from build123d import *

# Parameters (mm, degrees)
SKETCH_1_W           = 25.4
SKETCH_1_H           = 25.4
EXTRUDE_1_DEPTH      = 400.8
SKETCH_1_3_W         = 21.4
SKETCH_1_3_H         = 21.4
CUT_EXTRUDE_1_DEPTH  = 402.202218339
SKETCH_2_R           = 2.15
CUT_EXTRUDE_2_DEPTH  = 3
SKETCH_3_R           = 2.15
CUT_EXTRUDE_3_DEPTH  = 3
SKETCH_4_R           = 2.15
CUT_EXTRUDE_4_DEPTH  = 3
SKETCH_5_R           = 2.149999993
CUT_EXTRUDE_5_DEPTH  = 5
SKETCH_6_R           = 2.15
CUT_EXTRUDE_6_DEPTH  = 5
SKETCH_7_R           = 2.15
CUT_EXTRUDE_7_DEPTH  = 5
SKETCH_8_R           = 2.15
CUT_EXTRUDE_8_DEPTH  = 5
SKETCH_9_R           = 2.15
CUT_EXTRUDE_9_DEPTH  = 5
SKETCH_10_R          = 2.15
CUT_EXTRUDE_10_DEPTH = 5
SKETCH_12_R          = 2.15
CUT_EXTRUDE_11_DEPTH = 5
SKETCH_13_R          = 2.15
CUT_EXTRUDE_12_DEPTH = 5
SKETCH_14_R          = 2.15
CUT_EXTRUDE_13_DEPTH = 5
SKETCH_15_R          = 2.15
CUT_EXTRUDE_14_DEPTH = 5
SKETCH_16_R          = 2.5
CUT_EXTRUDE_15_DEPTH = 10
SKETCH_17_R          = 2.5
CUT_EXTRUDE_16_DEPTH = 10


with BuildPart() as part:
    # Sketch 1 → Extrude 1 (new body)
    with BuildSketch(Plane.XY):
        Rectangle(SKETCH_1_W, SKETCH_1_H)
    extrude(amount=EXTRUDE_1_DEPTH)

    # Sketch 1_3 → Cut-Extrude 1 (cut, through all)
    with BuildSketch(Plane.XY):
        Rectangle(SKETCH_1_3_W, SKETCH_1_3_H)
    extrude(amount=CUT_EXTRUDE_1_DEPTH, mode=Mode.SUBTRACT)

    # Sketch 2 → Cut-Extrude 2 (cut)
    with BuildSketch(Plane(origin=(12.7, 0, 0), x_dir=(0, 0, -1), z_dir=(1, 0, 0))):
        with Locations(Location((-43.1, 0, 0), (0, 0, 90))):
            Circle(SKETCH_2_R)
        with Locations(Location((-67.6, 0, 0), (0, 0, 90))):
            Circle(SKETCH_2_R)
    extrude(amount=-CUT_EXTRUDE_2_DEPTH, mode=Mode.SUBTRACT)

    # Sketch 3 → Cut-Extrude 3 (cut)
    with BuildSketch(Plane.XZ.offset(12.7)):
        with Locations(Location((0, 43.1, 0), (0, 0, 270))):
            Circle(SKETCH_3_R)
        with Locations(Location((0, 67.6, 0), (0, 0, 270))):
            Circle(SKETCH_3_R)
    extrude(amount=-CUT_EXTRUDE_3_DEPTH, mode=Mode.SUBTRACT)

    # Sketch 4 → Cut-Extrude 4 (cut)
    with BuildSketch(Plane(origin=(12.7, 0, 0), x_dir=(0, 0, -1), z_dir=(1, 0, 0))):
        with Locations(Location((-104.95, 0, 0), (0, 0, 90))):
            Circle(SKETCH_4_R)
    extrude(amount=-CUT_EXTRUDE_4_DEPTH, mode=Mode.SUBTRACT)

    # Sketch 5 → Cut-Extrude 5 (cut)
    with BuildSketch(Plane.XZ.offset(12.7)):
        with Locations(Location((0, 104.95, 0), (0, 0, 270))):
            Circle(SKETCH_5_R)
    extrude(amount=-CUT_EXTRUDE_5_DEPTH, mode=Mode.SUBTRACT)

    # Sketch 6 → Cut-Extrude 6 (cut)
    with BuildSketch(Plane(origin=(12.7, 0, 0), x_dir=(0, 0, -1), z_dir=(1, 0, 0))):
        with Locations(Location((-141.100000024, 0, 0), (0, 0, 90))):
            Circle(SKETCH_6_R)
    extrude(amount=-CUT_EXTRUDE_6_DEPTH, mode=Mode.SUBTRACT)

    # Sketch 7 → Cut-Extrude 7 (cut)
    with BuildSketch(Plane.XZ.offset(12.7)):
        with Locations(Location((0, 141.100000023, 0), (0, 0, 270))):
            Circle(SKETCH_7_R)
    extrude(amount=-CUT_EXTRUDE_7_DEPTH, mode=Mode.SUBTRACT)

    # Sketch 8 → Cut-Extrude 8 (cut)
    with BuildSketch(Plane.XZ.offset(12.7)):
        with Locations(Location((4.9, 133.3, 0), (0, 0, 270))):
            Circle(SKETCH_8_R)
        with Locations(Location((4.9, 162.75, 0), (0, 0, 270))):
            Circle(SKETCH_8_R)
    extrude(amount=-CUT_EXTRUDE_8_DEPTH, mode=Mode.SUBTRACT)

    # Sketch 9 → Cut-Extrude 9 (cut)
    with BuildSketch(Plane.XZ.offset(12.7)):
        with Locations(Location((0, 154.95, 0), (0, 0, 270))):
            Circle(SKETCH_9_R)
    extrude(amount=-CUT_EXTRUDE_9_DEPTH, mode=Mode.SUBTRACT)

    # Sketch 10 → Cut-Extrude 10 (cut)
    with BuildSketch(Plane(origin=(12.7, 0, 0), x_dir=(0, 0, -1), z_dir=(1, 0, 0))):
        with Locations(Location((-154.95, 0, 0), (0, 0, 90))):
            Circle(SKETCH_10_R)
    extrude(amount=-CUT_EXTRUDE_10_DEPTH, mode=Mode.SUBTRACT)

    # Sketch 12 → Cut-Extrude 11 (cut)
    with BuildSketch(Plane(origin=(12.7, 0, 0), x_dir=(0, 0, -1), z_dir=(1, 0, 0))):
        with Locations(Location((-133.3, -4.9, 0), (0, 0, 90))):
            Circle(SKETCH_12_R)
        with Locations(Location((-162.75, -4.9, 0), (0, 0, 90))):
            Circle(SKETCH_12_R)
    extrude(amount=-CUT_EXTRUDE_11_DEPTH, mode=Mode.SUBTRACT)

    # Sketch 13 → Cut-Extrude 12 (cut)
    with BuildSketch(Plane(origin=(12.7, 0, 0), x_dir=(0, 0, -1), z_dir=(1, 0, 0))):
        with Locations(Location((-179.55, 0, 0), (0, 0, 90))):
            Circle(SKETCH_13_R)
        with Locations(Location((-261.75, 0, 0), (0, 0, 90))):
            Circle(SKETCH_13_R)
    extrude(amount=-CUT_EXTRUDE_12_DEPTH, mode=Mode.SUBTRACT)

    # Sketch 14 → Cut-Extrude 13 (cut)
    with BuildSketch(Plane(origin=(12.7, 0, 0), x_dir=(0, 0, -1), z_dir=(1, 0, 0))):
        with Locations(Location((-193.100000003, 0, 0), (0, 0, 90))):
            Circle(SKETCH_14_R)
        with Locations(Location((-217.600000003, 0, 0), (0, 0, 90))):
            Circle(SKETCH_14_R)
    extrude(amount=-CUT_EXTRUDE_13_DEPTH, mode=Mode.SUBTRACT)

    # Sketch 15 → Cut-Extrude 14 (cut)
    with BuildSketch(Plane.XZ.offset(12.7)):
        with Locations(Location((-8e-09, 193.099999997, 0), (0, 0, 270))):
            Circle(SKETCH_15_R)
        with Locations(Location((-8e-09, 217.599999997, 0), (0, 0, 270))):
            Circle(SKETCH_15_R)
    extrude(amount=-CUT_EXTRUDE_14_DEPTH, mode=Mode.SUBTRACT)

    # Sketch 16 → Cut-Extrude 15 (cut)
    with BuildSketch(Plane(origin=(0, 12.7, 0), x_dir=(1, 0, 0), z_dir=(0, 1, 0))):
        with Locations(Location((0, -240.48, 0), (0, 0, 270))):
            Circle(SKETCH_16_R)
        with Locations(Location((0, -320.64, 0), (0, 0, 270))):
            Circle(SKETCH_16_R)
        with Locations(Location((0, -160.32, 0), (0, 0, 270))):
            Circle(SKETCH_16_R)
        with Locations(Location((0, -80.16, 0), (0, 0, 270))):
            Circle(SKETCH_16_R)
    extrude(amount=-CUT_EXTRUDE_15_DEPTH, mode=Mode.SUBTRACT)

    # Sketch 17 → Cut-Extrude 16 (cut)
    with BuildSketch(Plane.ZY.offset(12.7)):
        with Locations(Location((80.16, 0, 0), (0, 0, 270))):
            Circle(SKETCH_17_R)
        with Locations(Location((160.32, 0, 0), (0, 0, 270))):
            Circle(SKETCH_17_R)
        with Locations(Location((240.48, 0, 0), (0, 0, 270))):
            Circle(SKETCH_17_R)
        with Locations(Location((320.64, 0, 0), (0, 0, 270))):
            Circle(SKETCH_17_R)
    extrude(amount=-CUT_EXTRUDE_16_DEPTH, mode=Mode.SUBTRACT)


solid = part.part
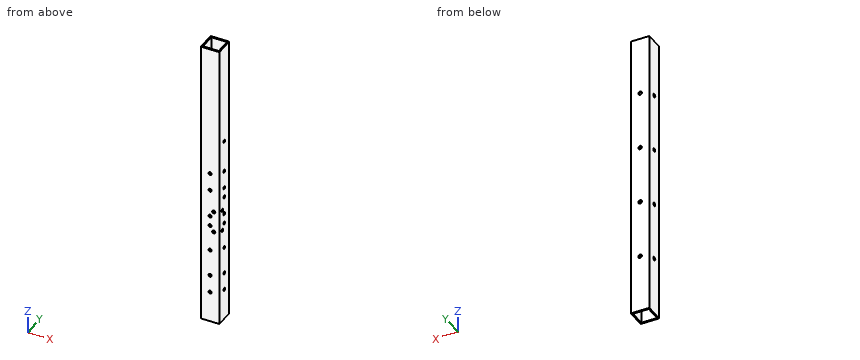
Source: CAD feature listing. Evaluate the final solid. Frame: model axes, mm. Round coordinates to 2 decimals unless told otherwise and drop trailing zeros. Loops run counter-clockwise (first coordinate to the right, second up) from the corner with the lowest first, then second, coordinate; pieces in that order, holes last.
Q1. Ray query, line 1 (Y direction, x = 8, z = 336.5); line 2 (Y direction, x = -11.35, z = 320.64). Return the intervals inside material, ascending.
Q2. First-contact query: P1, Ø4, axis at x = -8, y = 8.5, coming from the +Z side; P2, Ø3, axis at x = 0, z = 320.64, coming from the +Y side; P3, Ø4, axis at y = 0, z = 179.55, coming from the +X side. Flat tips, straight axial feed; report the tip coordinate or a pass-through.
Q3. Section A-A, the plane y = 6. Return loops of the section in (x, z).
Q4. Section C-C, the plane z = 29. Return loops of the section in (x, y), plus the area to 3 significant figures.
Solutions:
1. line 1: y = -12.7 to -10.7, 10.7 to 12.7
1. line 2: y = -12.7 to -2.5, 2.5 to 12.7
2. P1: passes through
2. P2: stops at y = -10.7
2. P3: stops at x = -10.7
3. outline: (-12.7, 0) - (-10.7, 0) - (-10.7, 400.8) - (-12.7, 400.8) - close; (10.7, 0) - (12.7, 0) - (12.7, 400.8) - (10.7, 400.8) - close
4. outline: (-12.7, -12.7) - (12.7, -12.7) - (12.7, 12.7) - (-12.7, 12.7) - close; hole (-10.7, -10.7) - (10.7, -10.7) - (10.7, 10.7) - (-10.7, 10.7) - close
4. area: 187 mm2
